Source: CAD feature listing. Evaluate the final solid. Frame: model axes, mm. A direction names the side the tool comes from. Give positions to 0.01 mm unless a question says otherwise; leave off trailing zeros. Loops run counter-clockwise (first coordinate to the right, second up) from the corner with the lowest first, then second, coordinate; pieces in that order, holes last. Notation, with made-up numbers: M -1,83 L 51,83 A24 cw 51,97 Z; hole C 78,6.25 d11. An arc over 180 degrees is marked long. Put each result on its own line as item: value.
from build123d import *

# Parameters (mm, degrees)
BOSS_EXTRUDE2_DEPTH = 3.5
SKETCH3_R           = 2.5
BOSS_EXTRUDE3_DEPTH = 5
FILLET2_R           = 0.5
SKETCH5_R           = 0.5
CUT_EXTRUDE1_DEPTH  = 1
SKETCH6_R           = 1
CUT_EXTRUDE2_DEPTH  = 6


with BuildPart() as part:
    # Sketch2 → Boss-Extrude2 (new body)
    with BuildSketch(Plane(origin=(0, 0, 0), x_dir=(1, 0, 0), z_dir=(0, 1, 0))):
        with BuildLine():
            Line((-1.500662684, 17.128376176), (-1.500662684, 12.128376176))
            Line((-1.500662684, 12.128376176), (2.499337316, 12.128376176))
            Line((2.499337316, 12.128376176), (2.499337316, 14.162218976))
            ThreePointArc((2.499337316, 14.162218976), (2.696087031, 14.75786063), (3.208915276, 15.119117632))
            Line((3.208915276, 15.119117632), (13.789759356, 18.330440279))
            ThreePointArc((13.789759356, 18.330440279), (14.302587601, 18.691697281), (14.499337316, 19.287338935))
            Line((14.499337316, 19.287338935), (14.499337316, 27.287338935))
            Line((14.499337316, 27.287338935), (15.499337316, 28.444539704))
            Line((15.499337316, 28.444539704), (15.499337316, 28.878255261))
            Line((15.499337316, 28.878255261), (15.499337316, 31.444539704))
            Line((15.499337316, 31.444539704), (10.499337316, 31.444539704))
            Line((10.499337316, 31.444539704), (10.499337316, 26.210120497))
            Line((10.499337316, 26.210120497), (10.499337316, 22.253496135))
            ThreePointArc((10.499337316, 22.253496135), (10.302587601, 21.657854481), (9.789759356, 21.296597478))
            Line((9.789759356, 21.296597478), (-0.791084724, 18.085274832))
            ThreePointArc((-0.791084724, 18.085274832), (-1.303912969, 17.724017829), (-1.500662684, 17.128376176))
        make_face()
    extrude(amount=BOSS_EXTRUDE2_DEPTH)

    # Sketch3 → Boss-Extrude3 (add)
    with BuildSketch(Plane.ZY.offset(-10.499337316)):
        with Locations((-31.444539704, 1.75)):
            Circle(SKETCH3_R)
    extrude(amount=-BOSS_EXTRUDE3_DEPTH)

    # Fillet2
    fillet2_edges = [part.edges().sort_by_distance(p)[0] for p in [
        (15.499337316, 1.75, -28.444539704),
        (14.499337316, 1.75, -27.287338935),
    ]]
    fillet(fillet2_edges, radius=FILLET2_R)

    # Sketch5 → Cut-Extrude1 (cut)
    with BuildSketch(Plane.XY.offset(-12.128376176)):
        with Locations((0.499337316, 1.75)):
            Circle(SKETCH5_R)
    extrude(amount=-CUT_EXTRUDE1_DEPTH, mode=Mode.SUBTRACT)

    # Sketch6 → Cut-Extrude2 (cut, through all)
    with BuildSketch(Plane.ZY.offset(-10.499337316)):
        with Locations((-31.444539704, 1.75)):
            Circle(SKETCH6_R)
    extrude(amount=-CUT_EXTRUDE2_DEPTH, mode=Mode.SUBTRACT)


solid = part.part
1. Contact query for flat-ended pins moving along their axis: P1, Ø0.6, axis at y = 2, z = -13.5, coming from the +X side; P2, Ø2, axis at x = 8, z = -30.5, coming from the -Y side; P3, Ø1, axis at x = 5.5, y = 2, coming from the +Z side; P4, Ø2.5, axis at y = 1.75, z = -31.44, coming from the -X side. Output: stop coordinate, or through.
Found:
P1: x = 2.5
P2: through
P3: z = -15.66
P4: x = 10.5
2. Section query C-C (z = -23.5). Output: boundary loops of the cut face in (x, y).
Found:
outline: M 10.5,0 L 14.5,0 L 14.5,3.5 L 10.5,3.5 Z
3. Material intervals for line 1 (Y direction, x = 12, z = -20.25); line 2 (Z direction, x = 12.75, y = 1.7); line 3 (X direction, y = 3.45, z = -32.5), sorted ascending. Write a range as from..to.
Found:
line 1: 0..3.5
line 2: -33.94..-32.44, -30.45..-18.01
line 3: 10.5..15.5
4. Section query D-D (y = 3.2). Output: boundary loops of the cut face in (x, z).
Found:
outline: M -1.5,-17.13 A1 ccw -0.79,-18.09 L 9.79,-21.3 A1 cw 10.5,-22.25 L 10.5,-33.48 L 15.5,-33.48 L 15.5,-28.63 A0.5 ccw 15.38,-28.3 L 14.62,-27.43 A0.5 cw 14.5,-27.1 L 14.5,-19.29 A1 ccw 13.79,-18.33 L 3.21,-15.12 A1 cw 2.5,-14.16 L 2.5,-12.13 L -1.5,-12.13 Z
5. Section query A-A (y = 1.75). Output: boundary loops of the cut face in (x, z), plus the area to 3 significant figures.
Found:
outline: M -1.5,-17.13 A1 ccw -0.79,-18.09 L 9.79,-21.3 A1 cw 10.5,-22.25 L 10.5,-30.44 L 15.5,-30.44 L 15.5,-28.63 A0.5 ccw 15.38,-28.3 L 14.62,-27.43 A0.5 cw 14.5,-27.1 L 14.5,-19.29 A1 ccw 13.79,-18.33 L 3.21,-15.12 A1 cw 2.5,-14.16 L 2.5,-12.13 L 1,-12.13 L 1,-13.13 L 0,-13.13 L 0,-12.13 L -1.5,-12.13 Z; M 10.5,-33.94 L 15.5,-33.94 L 15.5,-32.44 L 10.5,-32.44 Z
area: 118 mm^2
6. Section query B-B (z = -32). Output: boundary loops of the cut face in (x, y), plus the area to 3 significant figures.
Found:
outline: M 10.5,-0.69 L 15.5,-0.69 L 15.5,0.92 L 10.5,0.92 Z; M 10.5,2.58 L 15.5,2.58 L 15.5,4.19 L 10.5,4.19 Z
area: 16.1 mm^2
7. Draft query along Y for faces 5 (the cylindrical face through (0.77, 2.17, -12.62)), 6 (the cylindrical face through (12.964, 1.833, -33.943)), 7 (the flat face through (9, 3.5, -19)). Return one class per face: pulls with the +Y half, pulls with the -Y half, needs draft (parallel to the pull), parting line crosses it, or undercut.
Found:
face 5: undercut
face 6: parting line crosses it
face 7: pulls with the +Y half
8. Access query for faces 1 (the flat face through (0.5, 1.8, -13.128)), 2 (the flat face through (2.499, 2, -13)), 3 (the flat face through (9, 0, -19)), 4 (the flat face through (10.499, 2, -28)). Directions: +Z, -Z, +X, -X, +Y, -Y. A direction counts if a zero-diameter tool reaches every point of the face in a straight line with its end or side. Return the directions, or none.
Found:
face 1: +Z
face 2: +Z, +X, +Y, -Y
face 3: +Z, +X, -X, -Y
face 4: -Z, -X, +Y, -Y
